from build123d import *

# Parameters (mm, degrees)
F1_DEPTH = 20
F2_SIZE  = 0.5


with BuildPart() as f1:
    # F0 (on Top) → F1 (new body)
    with BuildSketch(Plane.XY):
        with BuildLine():
            Line((9.95, 2.5), (-9.95, 2.5))
            Line((-9.95, 2.5), (-9.95, 0.75))
            Line((-9.95, 0.75), (-9.95, 0))
            Line((-9.95, 0), (-9.95, -0.75))
            Line((-9.95, -0.75), (-9.95, -2.5))
            Line((-9.95, -2.5), (9.95, -2.5))
            Line((9.95, -2.5), (9.95, -0.8))
            Line((9.95, -0.8), (8.5989125293, -0.8))
            ThreePointArc((8.5989125293, -0.8), (6.05, 0), (8.5989125293, 0.8))
            Line((8.5989125293, 0.8), (9.95, 0.8))
            Line((9.95, 0.8), (9.95, 2.5))
        make_face()
        with BuildLine():
            Line((-9.95, 0), (-9.95, 0.75))
            Line((-9.95, 0.75), (-11.327502784, 0.75))
            ThreePointArc((-11.327502784, 0.75), (-11.158127088, 0.391872912), (-11.1, 0))
            Line((-11.1, 0), (-9.95, 0))
        make_face()
        with BuildLine():
            ThreePointArc((-11.327502784, -0.75), (-11.158127088, -0.391872912), (-11.1, 0))
            Line((-11.1, 0), (-12.45, 0))
            Line((-12.45, 0), (-12.45, -0.75))
            Line((-12.45, -0.75), (-11.327502784, -0.75))
        make_face()
        with BuildLine():
            Line((-9.95, -0.75), (-9.95, 0))
            Line((-9.95, 0), (-11.1, 0))
            ThreePointArc((-11.1, 0), (-11.158127088, -0.391872912), (-11.327502784, -0.75))
            Line((-11.327502784, -0.75), (-9.95, -0.75))
        make_face()
        with BuildLine():
            Line((-12.45, 0.75), (-11.327502784, 0.75))
            ThreePointArc((-11.327502784, 0.75), (-13.8, 0), (-11.327502784, -0.75))
            Line((-11.327502784, -0.75), (-12.45, -0.75))
            Line((-12.45, -0.75), (-12.45, 0))
            Line((-12.45, 0), (-12.45, 0.75))
        make_face()
        with BuildLine():
            ThreePointArc((-11.1, 0), (-11.158127088, 0.391872912), (-11.327502784, 0.75))
            Line((-11.327502784, 0.75), (-12.45, 0.75))
            Line((-12.45, 0.75), (-12.45, 0))
            Line((-12.45, 0), (-11.1, 0))
        make_face()
    extrude(amount=F1_DEPTH)

    # F2
    f2_edges = [f1.edges().sort_by_distance(p)[0] for p in [
        (0, -2.5, 20),
        (-9.95, -1.625, 20),
        (-10.638751, -0.75, 20),
        (-13.8, 0, 20),
        (-10.638751, 0.75, 20),
        (-9.95, 1.625, 20),
        (0, 2.5, 20),
        (9.95, 1.65, 20),
        (9.274456, 0.8, 20),
        (6.05, 0, 20),
        (9.274456, -0.8, 20),
        (9.95, -1.65, 20),
        (9.95, -2.5, 10),
        (9.95, 2.5, 10),
        (-9.95, -2.5, 10),
        (-9.95, 2.5, 10),
        (0, -2.5, 0),
        (9.95, -1.65, 0),
        (9.274456, -0.8, 0),
        (6.05, 0, 0),
        (9.274456, 0.8, 0),
        (9.95, 1.65, 0),
        (0, 2.5, 0),
        (-9.95, 1.625, 0),
        (-10.638751, 0.75, 0),
        (-10.638751, -0.75, 0),
        (-9.95, -1.625, 0),
        (-13.8, 0, 0),
    ]]
    chamfer(f2_edges, length=F2_SIZE)


solid = f1.part
Could you check a few things on this model? Use its own coordinates, in mm. A direction names the side the tool comes from. Round coordinates to 2 decimals unless told otherwise and drop trailing zeros. Write each loop counter-clockwise with the first axis right and the second up, starting at its lowest first coordinate (ties: lowest second). Pieces come first, ordered by that corner, then holes. Notation, with made-up numbers: (28.25, 22.25) - (71.25, 22.25) arc R32 ccw to (71.25, 54.25) - close; hole circle Ø6 at (15, 71.5). An arc over 180 degrees is marked (long way). Put each result on its own line as item: value. Start each with the question number.
(1) For faces 1 (the flat face through (9, 0.8, 10)), 2 (the flat face through (-11, 0.75, 10)), 3 (the flat face through (-9.95, -1, 10)), which set-ups out of +Z, -Z, +X, -X, +Y, -Y let a thin tool reach every point of the face, with its end or its side?
(2) I want a section at B-B, the plane z = 6.5. Please give me the cut outline in (x, y).
(3) I want a section at C-C, the plane x = -12.45. Please give me the cut outline in (y, z).
(4) I want a section at A-A, the plane x = 7.45. Please give me the cut outline in (y, z), plus the area to 3 significant figures.
(5) I need wall thicknesses on probe 1 along Y at (x, z) = (7.45, 11); probe 2 along X at (y, z) = (-1.1, 4.25); probe 3 along X at (y, z) = (0.9, 9). Which ranges of each line are inside material? Lowest first, please.
(6) Will these pins go through, and if not, where does the flat tip stop? pin 1 (1 mm diameter, centred on y = -1.5, z = 14, fed in from -X); pin 2 (1 mm diameter, centred on y = 1, z = 12, fed in from -X); pin 3 (2 mm diameter, centred on x = 7.45, y = 0, fed in from +Z); pin 4 (2 mm diameter, centred on x = -10.5, z = 18, fed in from +Y).
(7) Thinking about a two-plate mould opening in X: for faces 4 (the flat face through (9.95, -1, 10)), 5 (the flat face through (0, -2.5, 10)), 6 (the flat face through (-9.95, 1, 10)), which applies, released by +X, released by -X, zero draft, split by the parting line, or undercut?
Here are the results:
1. face 1: +Z, -Z, +X
1. face 2: +Z, -Z, +Y
1. face 3: +Z, -Z, -Y
2. outline: (-11.33, -0.75) - (-9.95, -0.75) - (-9.95, -2) - (-9.45, -2.5) - (9.45, -2.5) - (9.95, -2) - (9.95, -0.8) - (8.6, -0.8) arc R1.4 cw (long way) to (8.6, 0.8) - (9.95, 0.8) - (9.95, 2) - (9.45, 2.5) - (-9.45, 2.5) - (-9.95, 2) - (-9.95, 0.75) - (-11.33, 0.75) arc R1.35 ccw (long way) to start
3. outline: (-1.35, 0.5) - (-0.85, 0) - (0.85, 0) - (1.35, 0.5) - (1.35, 19.5) - (0.85, 20) - (-0.85, 20) - (-1.35, 19.5) - close
4. outline: (-2.5, 0.5) - (-2, 0) - (-1.9, 0) - (-1.4, 0.5) - (-1.4, 19.5) - (-1.9, 20) - (-2, 20) - (-2.5, 19.5) - close; (1.4, 0.5) - (1.9, 0) - (2, 0) - (2.5, 0.5) - (2.5, 19.5) - (2, 20) - (1.9, 20) - (1.4, 19.5) - close
4. area: 43.0 mm^2
5. probe 1: y = -2.5 to -1.4, 1.4 to 2.5
5. probe 2: x = -13.23 to -11.67, -9.95 to 6.58, 8.32 to 9.95
5. probe 3: x = -13.46 to -11.44, -9.95 to 6.38, 8.52 to 9.95
6. pin 1: stops at x = -13.36
6. pin 2: stops at x = -13.7
6. pin 3: passes through
6. pin 4: stops at y = 2.45
7. face 4: released by +X
7. face 5: zero draft
7. face 6: undercut
